from build123d import *

# Parameters (mm, degrees)
F0_W     = 100.584
F0_H     = 25.4
F1_DEPTH = 3.175
F0_W_2   = 106.934
F0_H_2   = 31.75
F2_DEPTH = 9.525
F3_W     = 103.759
F3_H     = 28.575
F3_W_2   = 100.584
F3_H_2   = 25.4
F4_DEPTH = 6.35
F5_R     = 2.54


with BuildPart() as f1:
    # F0 (on Top) → F1 (new body)
    with BuildSketch(Plane.XY):
        with Locations((50.292, 12.7)):
            Rectangle(F0_W, F0_H)
    extrude(amount=F1_DEPTH)

    # F0 (on Top) → F2 (join)
    with BuildSketch(Plane.XY):
        with Locations((50.292, 12.7)):
            Rectangle(F0_W_2, F0_H_2)
        with Locations((50.292, 12.7)):
            Rectangle(F0_W, F0_H, mode=Mode.SUBTRACT)
    extrude(amount=F2_DEPTH)

    # F3 (on face) → F4 (cut)
    with BuildSketch(Plane.XY.offset(9.525)):
        with Locations((50.292, 12.7)):
            Rectangle(F3_W, F3_H)
        with Locations((50.292, 12.7)):
            Rectangle(F3_W_2, F3_H_2, mode=Mode.SUBTRACT)
    extrude(amount=-F4_DEPTH, mode=Mode.SUBTRACT)

    # F5
    f5_edges = [f1.edges().sort_by_distance(p)[0] for p in [
        (-1.5875, 26.9875, 6.35),
        (-1.5875, -1.5875, 6.35),
        (102.1715, -1.5875, 6.35),
        (102.1715, 26.9875, 6.35),
        (-3.175, -3.175, 4.7625),
        (103.759, -3.175, 4.7625),
        (103.759, 28.575, 4.7625),
        (-3.175, 28.575, 4.7625),
    ]]
    fillet(f5_edges, radius=F5_R)


solid = f1.part
Model file for the job. Use its own axes, mm. A direction names the side the tool comes from. Give positions to 0.01 mm unless a question says otherwise; leave off trailing zeros. Loops run counter-clockwise (first coordinate to the right, second up) from the corner with the lowest first, then second, coordinate; pieces in that order, holes last.
1) Saw through at B-B (y = 11). Write the cut outline in (x, z) (1 decimal).
2) Saw through at C-C (x = 39). Write the cut outline in (y, z) (1 decimal), plus the area to 3 significant figures.
3) Saw through at A-A (z = 4.5). Write the cut outline in (x, y) (1 decimal).
4) Flat gauge pin, fed straight in: pin 1 Ø3 at (x, y) = (21.5, 19) entering from +Z (3 decimals). Where does the tip first touch, or does it go through?
5) Pull direction X, two halves, no side cores. Call faces 1 (the flat face through (50, 13, 0)), 2 (the flat face through (103.759, 13, 5)), 3 (the cylindrical face through (-2.45, 27.81, 4.83)), 4 (the flat face through (50, -1.588, 6)): +X half, -X half, draft (parallel to the pull), parting line (faces both ways), or undercut.
6) Tool access for faces 5 (the flat face through (50, 26.987, 6)), 6 (the flat face through (50, -3.175, 5)): list every direction of +Z, -Z, +X, -X, +Y, -Y with a clear straight run to the whole face (end or side of a thin tool).
7) Wall check: line 1 (Y direction, x = 58, z = 9) (1 decimal); line 2 (X direction, y = 11, z = 6.5) (1 decimal); line 3 (Z direction, x = 37, y = 15.5) (3 decimals). Give the ranges that are in metal, low to high.
Answer block:
1. outline: (-3.2, 0) - (103.8, 0) - (103.8, 9.5) - (102.2, 9.5) - (102.2, 3.2) - (-1.6, 3.2) - (-1.6, 9.5) - (-3.2, 9.5) - close
2. outline: (-3.2, 0) - (28.6, 0) - (28.6, 9.5) - (27, 9.5) - (27, 3.2) - (-1.6, 3.2) - (-1.6, 9.5) - (-3.2, 9.5) - close
2. area: 121 mm2
3. outline: (-3.2, -0.6) arc R2.5 ccw to (-0.6, -3.2) - (101.2, -3.2) arc R2.5 ccw to (103.8, -0.6) - (103.8, 26) arc R2.5 ccw to (101.2, 28.6) - (-0.6, 28.6) arc R2.5 ccw to (-3.2, 26) - close; hole (-1.6, 1) arc R2.5 ccw to (1, -1.6) - (99.6, -1.6) arc R2.5 ccw to (102.2, 1) - (102.2, 24.4) arc R2.5 ccw to (99.6, 27) - (1, 27) arc R2.5 ccw to (-1.6, 24.4) - close
4. pin 1: stops at z = 3.175
5. face 1: draft
5. face 2: +X half
5. face 3: -X half
5. face 4: undercut
6. face 5: +Z
6. face 6: +Z, -Z, +X, -X, -Y
7. line 1: y = -3.2 to -1.6, 27 to 28.6
7. line 2: x = -3.2 to -1.6, 102.2 to 103.8
7. line 3: z = 0 to 3.175
